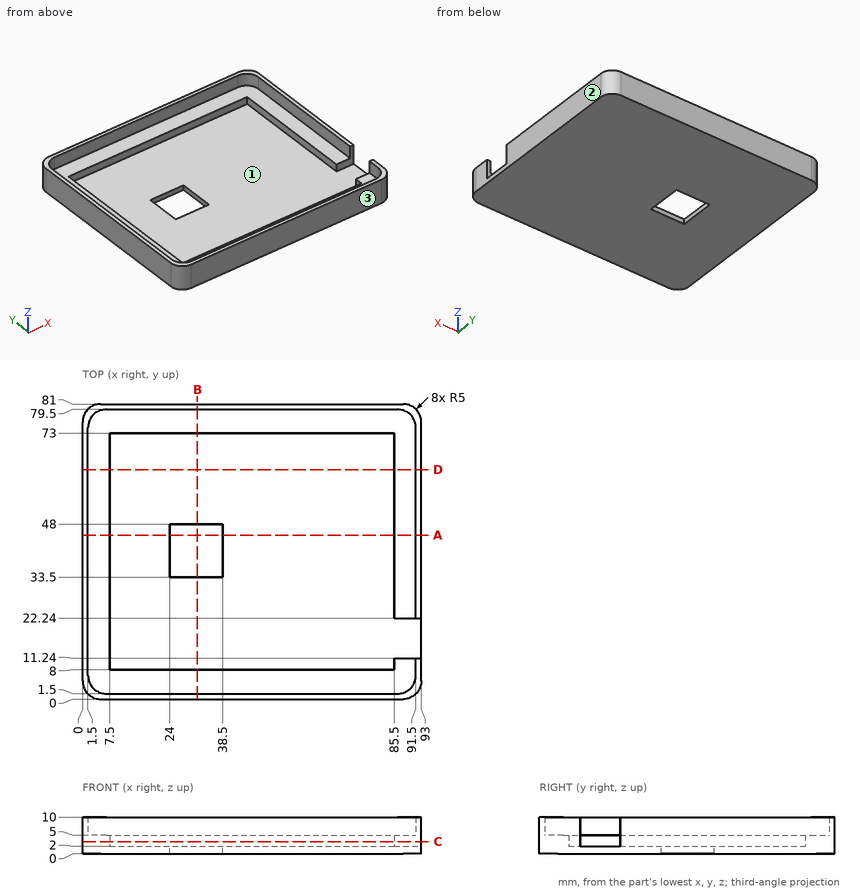
Here's the drawing with two shaded views (mm, measured from the low corner). I have some questions. Coordinates: 2 decimals unless noted, no trailing zeros. Write each loop counter-clockwise with the first axis right and the second up, starting at its lowest first coordinate (ties: lowest second). Pieces come first, ordered by that corner, then holes. Notation, with made-up numbers: (-33, 0.5) - (-4, 0.5) arc R26 ccw to (-4, 28.5) - close; hole circle Ø11 at (38, 88). An arc over 180 degrees is marked (long way). Return JSON: item names as keys, results as strings.
Q1. Please list where these lines run through material, in increasing order: L1, parallel to Y at x = 32, z = 8.5; L2, parallel to Y at x = 42.5, z = 4.25; L3, parallel to X at y = 45.5, z = 8.25. Write a range as from..to.
Computed values:
{"L1": "y = 0..1.5, 79.5..81", "L2": "y = 0..8, 73..81", "L3": "x = 0..1.5, 91.5..93"}
Q2. I'm going to push flat-ended pins straight in: pin 1 Ø5 at (x, y) = (46, 49.5) entering from +Z; pin 2 Ø2 at (x, y) = (62, 72.5) entering from +Z. Where does each tip first touch, or does it pass through?
Computed values:
{"pin 1": "stops at z = 2", "pin 2": "stops at z = 5"}
Q3. If we section it at A-A (y = 45): Please give me the cut outline in (x, z), then the cut area to 3 significant figures.
Computed values:
{"outline": "(0, 0) - (24, 0) - (24, 2) - (7.5, 2) - (7.5, 5) - (1.5, 5) - (1.5, 10) - (0, 10) - close; (38.5, 0) - (93, 0) - (93, 10) - (91.5, 10) - (91.5, 5) - (85.5, 5) - (85.5, 2) - (38.5, 2) - close", "area": "217 mm2"}
Q4. Thinking about a two-plate mould opening in Y: for the marked faces 1, 2 and 3, which applies, +Y half, -Y half, draft (parallel to the pull), parting line (faces both ways), or undercut?
Computed values:
{"face 1": "undercut", "face 2": "draft", "face 3": "-Y half"}
Q5. If we section it at C-C (z = 3.25): Please give me the cut outline in (x, y), then the cut area to 3 significant figures.
Computed values:
{"outline": "(0, 5) arc R5 ccw to (5, 0) - (88, 0) arc R5 ccw to (93, 5) - (93, 11.24) - (85.5, 11.24) - (85.5, 8) - (7.5, 8) - (7.5, 73) - (85.5, 73) - (85.5, 22.24) - (93, 22.24) - (93, 76) arc R5 ccw to (88, 81) - (5, 81) arc R5 ccw to (0, 76) - close", "area": "2,360 mm2"}
Q6. If we section it at D-D (y = 63): Please give me the cut outline in (x, z), then the cut area to 3 significant figures.
Computed values:
{"outline": "(0, 0) - (93, 0) - (93, 10) - (91.5, 10) - (91.5, 5) - (85.5, 5) - (85.5, 2) - (7.5, 2) - (7.5, 5) - (1.5, 5) - (1.5, 10) - (0, 10) - close", "area": "246 mm2"}
Q7. If we section it at B-B (x = 31.5): Please give me the cut outline in (y, z).
Computed values:
{"outline": "(0, 0) - (33.5, 0) - (33.5, 2) - (8, 2) - (8, 5) - (1.5, 5) - (1.5, 10) - (0, 10) - close; (48, 0) - (81, 0) - (81, 10) - (79.5, 10) - (79.5, 5) - (73, 5) - (73, 2) - (48, 2) - close"}
